from build123d import *

# Parameters (mm, degrees)
BOSS_EXTRUDE1_DEPTH = 87.5
SKETCH1_3_W         = 88
SKETCH1_3_H         = 40
BOSS_EXTRUDE2_DEPTH = 50
BOSS_EXTRUDE3_DEPTH = 16
FILLET1_RADIUS      = 37.5
FILLET1_LENGTH      = 88
CUT_EXTRUDE1_REACH  = 206.864
SKETCH4_R           = 25
SKETCH4_R_2         = 5.1


with BuildPart() as part:
    # Sketch1 → Boss-Extrude1 (new body)
    with BuildSketch(Plane(origin=(0, 0, 0), x_dir=(0, 0, -1), z_dir=(1, 0, 0))):
        Polygon((88, 40), (88, 0), (163, 0), (163, 88), (88, 88), align=None)
    extrude(amount=BOSS_EXTRUDE1_DEPTH)

    # Sketch1<3> → Boss-Extrude2 (add)
    with BuildSketch(Plane(origin=(0, 0, 0), x_dir=(0, 0, -1), z_dir=(1, 0, 0))):
        with Locations((44, 20)):
            Rectangle(SKETCH1_3_W, SKETCH1_3_H)
        with BuildLine():
            ThreePointArc((25, 9), (14, 20), (25, 31))
            Line((25, 31), (63, 31))
            ThreePointArc((63, 31), (74, 20), (63, 9))
            Line((63, 9), (25, 9))
        make_face(mode=Mode.SUBTRACT)
    extrude(amount=BOSS_EXTRUDE2_DEPTH)

    # Sketch1<4> → Boss-Extrude3 (add)
    with BuildSketch(Plane(origin=(0, 0, 0), x_dir=(0, 0, -1), z_dir=(1, 0, 0))):
        Polygon((88, 88), (0, 40), (88, 40), align=None)
    extrude(amount=BOSS_EXTRUDE3_DEPTH)

    # Fillet1: full round fillet: the end face becomes a half cylinder, R = half its width
    fillet1_face = Plane((87.5, 44, -125.5), x_dir=(0, 1, 0), z_dir=(1, 0, 0))  # on the end face: x along it, z out of the body
    fillet1_slab = fillet1_face.offset(-FILLET1_RADIUS / 2) * Box(FILLET1_LENGTH, 2 * FILLET1_RADIUS, FILLET1_RADIUS, mode=Mode.PRIVATE)  # the body's end, R deep
    fillet1_round = Plane((50, 44, -125.5), x_dir=(1, 0, 0), z_dir=(0, 1, 0)) * Cylinder(FILLET1_RADIUS, FILLET1_LENGTH, mode=Mode.PRIVATE)  # its axis R under the face
    add(fillet1_slab - fillet1_round, mode=Mode.SUBTRACT)

    # Sketch4 → Cut-Extrude1 (cut, up to next)
    with BuildSketch(Plane(origin=(0, 88, 0), x_dir=(1, 0, 0), z_dir=(0, 1, 0)), mode=Mode.PRIVATE) as cut_extrude1_sk1:
        with Locations(Location((50, 125.5, 0), (0, 0, 270))):
            Circle(SKETCH4_R)
    cut_extrude1_tool1 = extrude(cut_extrude1_sk1.sketch, amount=-CUT_EXTRUDE1_REACH, mode=Mode.PRIVATE) & part.part
    # Sketch4 → Cut-Extrude1 (cut, up to next)
    with BuildSketch(Plane(origin=(0, 88, 0), x_dir=(1, 0, 0), z_dir=(0, 1, 0)), mode=Mode.PRIVATE) as cut_extrude1_sk2:
        with Locations(Location((33, 44, 0), (0, 0, 270))):
            Circle(SKETCH4_R_2)
    cut_extrude1_tool2 = extrude(cut_extrude1_sk2.sketch, amount=-CUT_EXTRUDE1_REACH, mode=Mode.PRIVATE) & part.part
    add(cut_extrude1_tool1.solids().sort_by_distance((50, 88, -125.5))[0], mode=Mode.SUBTRACT)
    add(cut_extrude1_tool2.solids().sort_by_distance((33, 88, -44))[0], mode=Mode.SUBTRACT)


solid = part.part
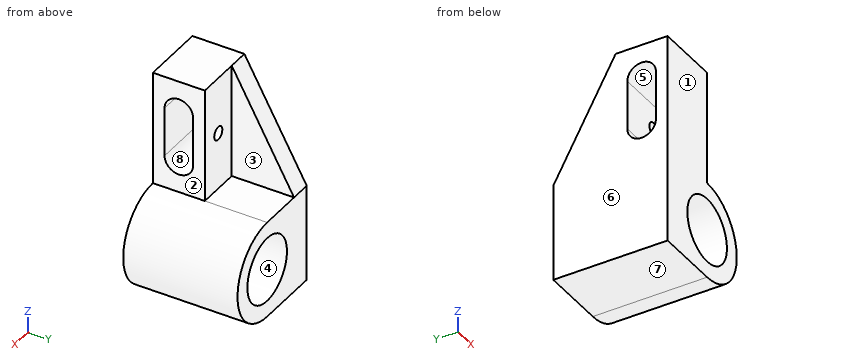
The model under review builds one solid part; all positions refer to its coordinate system, in mm. Face numbers are marked on the shaded views. A direction names the side the tool comes from. Round coordinates to 2 decimals unless told otherwise and drop trailing zeros. Loops run counter-clockwise (first coordinate to the right, second up) from the corner with the lowest first, then second, coordinate; pieces in that order, holes last. Notation, with made-up numbers: (-5.5, -20) -> (3.5, -20) arc R28 cw to (3.5, 9) -> close; hole circle Ø1 at (38.25, 77.25). An arc over 180 degrees is marked (long way). Answer as CSV lines item,"result".
1) Tool access review of the marked faces 1, 2, 3, 4 and 5: name each direction out of +Z, -Z, +X, -X, +Y, -Y from which nothing blocks a thin tool from reaching the whole face with its end or side.
Geometry results:
face 1,"+Z, -Z, +X, -X, -Y"
face 2,"+Z, +X, +Y, -Y"
face 3,"+Z, +X, +Y"
face 4,"+Y, -Y"
face 5,"+X, -X"
2) Draft analysis for pull direction Z (two halves, no side actions). For the marked faces 6, 7 and 8, state which applies: pulls with the +Z half, pulls with the -Z half, needs draft (parallel to the pull), parting line crosses it, or undercut.
Geometry results:
face 6,"needs draft"
face 7,"pulls with the -Z half"
face 8,"undercut"
3) Add section B-B on y = 20. Write out the cut boundary in (x, z), plus the area to 3 significant figures.
Geometry results:
outline,"(0, -163) -> (50, -163) arc R37.5 ccw to (50, -88) -> (50, -74) -> (0, -74) -> close; (0, -14) -> (50, -14) -> (50, 0) -> (0, 0) -> close; hole circle Ø50 at (50, -125.5)"
area,"5,400 mm²"
4) Add section C-C on x = 12. Write out the cut boundary in (y, z), plus the area to 3 significant figures.
Geometry results:
outline,"(0, -163) -> (88, -163) -> (88, -88) -> (40, 0) -> (0, 0) -> close; hole (9, -63) arc R11 ccw to (31, -63) -> (31, -25) arc R11 ccw to (9, -25) -> close"
area,"11,000 mm²"
5) For P1, Ø24, axis at y = 75.5, z = -61, coming from the +X side; P2, Ø13.5, axis at x = 33, z = -44, coming from the +Y side; P3, Ø5, axis at x = 69.5, y = 66, coming from the -Z side, all flat-tipped, find the tip position at first contact; note any pin that passes through.
Geometry results:
P1,"stops at x = 16"
P2,"stops at y = 40"
P3,"stops at z = -158.93"
6) Add section D-D on y = 33. Write out the cut boundary in (x, z).
Geometry results:
outline,"(0, -163) -> (50, -163) arc R37.5 ccw to (50, -88) -> (50, 0) -> (0, 0) -> close; hole circle Ø50 at (50, -125.5); hole circle Ø10.2 at (33, -44)"
7) To check wall thickness, follow line 1 along X through (y, z) = (24.5, -125.5); line 2 along X through (y, z) = (33.25, -44); line 3 along Z through (x, y) = (71.5, 58). State the ranges of each line that lie inside material, in increasing order. Write a range as from..to.
Geometry results:
line 1,"x = 0..25, 75..87.5"
line 2,"x = 0..27.9, 38.1..50"
line 3,"z = -156.22..-138.26, -112.74..-94.78"
8) Add section A-A on z = -44. Write out the cut boundary in (x, y).
Geometry results:
outline,"(0, 0) -> (50, 0) -> (50, 9) -> (0, 9) -> close; (0, 31) -> (27.9, 31) -> (27.9, 40) -> (16, 40) -> (16, 64) -> (0, 64) -> close; (38.1, 31) -> (50, 31) -> (50, 40) -> (38.1, 40) -> close"
